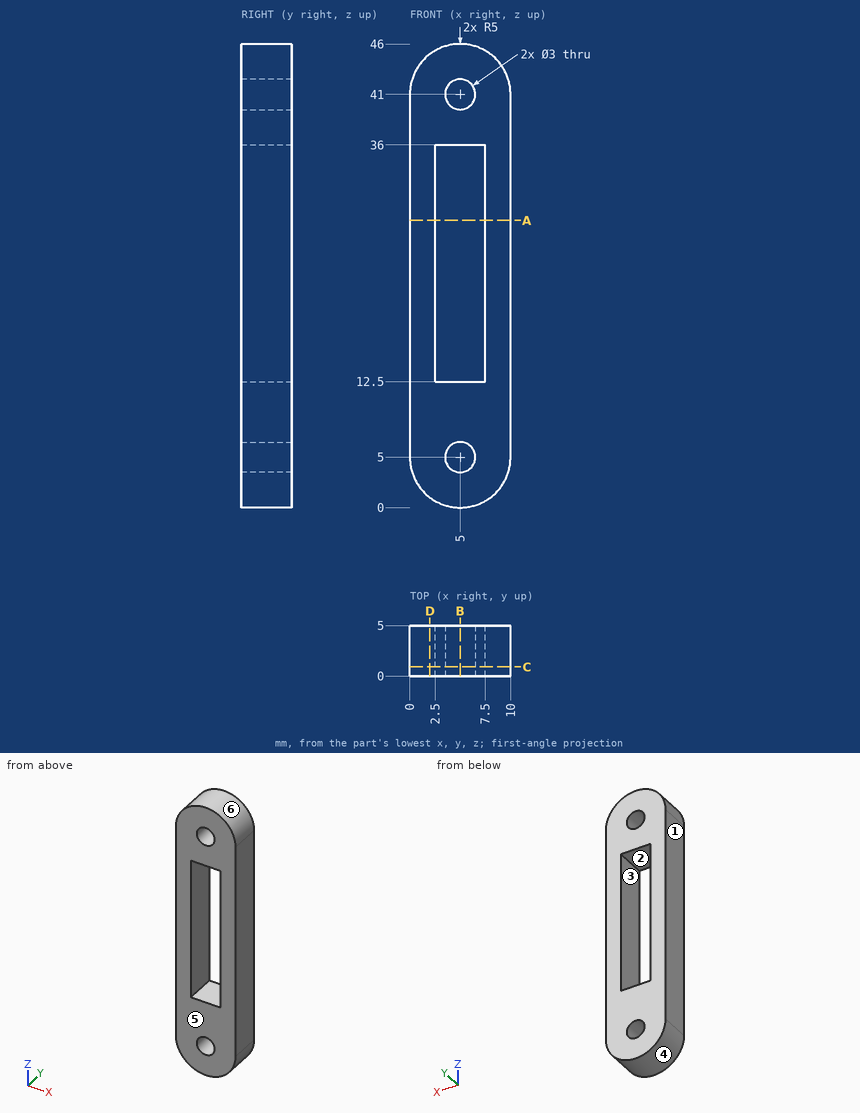
The figure shows three views and two pictorial views of one solid part (mm, origin at its lowest corner). Answer the questions. A direction names the side the tool comes from. Give positions to 0.01 mm unless a question says otherwise; leave off trailing zeros. Write each loop counter-clockwise with the first axis right and the second up, starting at its lowest first coordinate (ties: lowest second). Pieces come first, ordered by that corner, then holes. Notation, with made-up numbers: (78.25, 0.5) -> (108.25, 0.5) arc R31 ccw to (108.25, 25.5) -> close; hole circle Ø6 at (78, 9.5). An arc over 180 degrees is marked (long way). Answer as a JSON object with one key per item and string values.
1) A tool of negligible diameter and unlimited length cuts with its end or side. For the marked faces 1 and 2, from which of +Z, -Z, +X, -X, +Y, -Y can it reach the whole face along a straight path? Write none if from no direction.
Findings below:
{"face 1": "+Z, -Z, -X, +Y, -Y", "face 2": "+Y, -Y"}
2) Section B-B on x = 5 is taken. Write down the section's boundary in (y, z), then the cut area to 3 significant figures.
Findings below:
{"outline": "(0, 0) -> (5, 0) -> (5, 3.5) -> (0, 3.5) -> close; (0, 6.5) -> (5, 6.5) -> (5, 12.5) -> (0, 12.5) -> close; (0, 36) -> (5, 36) -> (5, 39.5) -> (0, 39.5) -> close; (0, 42.5) -> (5, 42.5) -> (5, 46) -> (0, 46) -> close", "area": "82.5 mm^2"}
3) Straight lines are drawn through the part: probe 1 along Z at (x, y) = (4.5, 1.4); probe 2 along X at (y, z) = (3.05, 5); probe 3 along X at (y, z) = (0.45, 29). For each, find the intervals that lie inside material, in ascending order. Write a range as from..to.
Findings below:
{"probe 1": "z = 0.03..3.59, 6.41..12.5, 36..39.59, 42.41..45.97", "probe 2": "x = 0..3.5, 6.5..10", "probe 3": "x = 0..2.5, 7.5..10"}
4) Section C-C on y = 0.9 is taken. Write down the section's boundary in (x, z), then the cut area to 3 significant figures.
Findings below:
{"outline": "(0, 5) arc R5 ccw to (10, 5) -> (10, 41) arc R5 ccw to (0, 41) -> close; hole (2.5, 12.5) -> (7.5, 12.5) -> (7.5, 36) -> (2.5, 36) -> close; hole circle Ø3 at (5, 5); hole circle Ø3 at (5, 41)", "area": "307 mm^2"}
5) Section D-D on x = 2 is taken. Write down the section's boundary in (y, z), then the cut area to 3 significant figures.
Findings below:
{"outline": "(0, 1) -> (5, 1) -> (5, 45) -> (0, 45) -> close", "area": "220 mm^2"}
6) For a pull along Z with two mould halves and no side action, classify the marked faces 3, 4, 5 and 6 as pulls with the +Z half, pulls with the -Z half, needs draft (parallel to the pull), parting line crosses it, or undercut.
Findings below:
{"face 3": "undercut", "face 4": "pulls with the -Z half", "face 5": "needs draft", "face 6": "pulls with the +Z half"}
7) Section A-A on z = 28.5 is taken. Write down the section's boundary in (x, y).
Findings below:
{"outline": "(0, 0) -> (2.5, 0) -> (2.5, 5) -> (0, 5) -> close; (7.5, 0) -> (10, 0) -> (10, 5) -> (7.5, 5) -> close"}
8) A flat-ended cylindrical pin translates along its axis: pin 1 Ø2 at (x, y) = (3, 1) entering from -Z. Find the tip coordinate at first contact, or state that the pin passes through.
Findings below:
{"pin 1": "stops at z = 0.1"}
